from build123d import *

# Parameters (mm, degrees)
F0_W     = 273.05
F0_H     = 114.3
F1_DEPTH = 19.05
F2_R     = 25.4
F3_DEPTH = 25.4
F5_DEPTH = 25.4
F7_DEPTH = 25.4
F8_W     = 19.3382904482
F8_H     = 2.7599734166
F9_DEPTH = 25.4


# Not quite as in the source:
# - a feature names something its author has since deleted; it is built from what else it names


with BuildPart() as f1:
    # F0 (on Front) → F1 (new body)
    with BuildSketch(Plane.XZ):
        with Locations((136.525, 57.15)):
            Rectangle(F0_W, F0_H)
    extrude(amount=F1_DEPTH)

    # F2 (on face) → F3 (cut)
    with BuildSketch(Plane.XZ.offset(19.05)):
        with Locations((50.8, 47.625)):
            Circle(F2_R)
        with Locations((222.25, 47.625)):
            Circle(F2_R)
    extrude(amount=-F3_DEPTH, mode=Mode.SUBTRACT)

    # F4 (on face) → F5 (cut)
    with BuildSketch(Plane.XZ.offset(19.05)):
        with BuildLine():
            Line((200.0185036906, 35.3400265834), (73.0314963094, 35.3400265834))
            ThreePointArc((73.0314963094, 35.3400265834), (68.4136636998, 29.3242117364), (62.225616864, 24.9398665581))
            Line((62.225616864, 24.9398665581), (210.824383136, 24.9398665581))
            ThreePointArc((210.824383136, 24.9398665581), (204.6363363002, 29.3242117364), (200.0185036906, 35.3400265834))
        make_face()
    extrude(amount=-F5_DEPTH, mode=Mode.SUBTRACT)

    # F6 (on face) → F7 (cut)
    with BuildSketch(Plane.XZ.offset(19.05)):
        with BuildLine():
            Line((177.8, 114.3), (95.25, 114.3))
            Line((95.25, 114.3), (95.25, 49.53))
            ThreePointArc((95.25, 49.53), (98.597769491, 41.447769491), (106.68, 38.1))
            Line((106.68, 38.1), (166.37, 38.1))
            ThreePointArc((166.37, 38.1), (174.452230509, 41.447769491), (177.8, 49.53))
            Line((177.8, 49.53), (177.8, 114.3))
        make_face()
    extrude(amount=-F7_DEPTH, mode=Mode.SUBTRACT)

    # F8 (on face) → F9 (cut)
    with BuildSketch(Plane.XZ.offset(19.05)):
        with Locations((156.7008547759, 36.7200132917)):
            Rectangle(F8_W, F8_H)
    extrude(amount=-F9_DEPTH, mode=Mode.SUBTRACT)


solid = f1.part
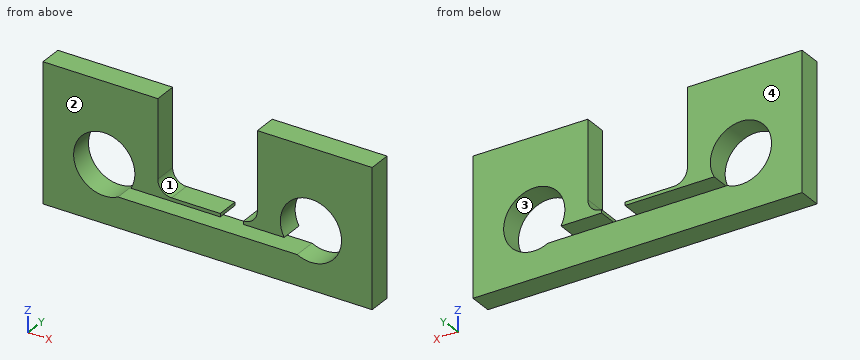
Design review of the part built by this model. Coordinates are the model's own, in mm. Face numbers are marked on the shaded views. A direction names the side the tool comes from. Give positions to 0.01 mm unless a question says otherwise; leave off trailing zeros. Write each loop counter-clockwise with the first axis right and the second up, starting at its lowest first coordinate (ties: lowest second). Pieces come first, ordered by that corner, then holes. Notation, with made-up numbers: M -32,22.25 L -2,22.25 A13 ccw -2,41.25 Z; hole C -23,5 d11. An arc over 180 degrees is marked long. Return JSON: item names as keys, results as strings. Group by question number.
Item 1: The part is to be moulded in two halves that separate along X. For the marked faces 3 and 4, say which applies: pulls with the +X half, pulls with the -X half, needs draft (parallel to the pull), parting line crosses it, or undercut.
Item 2: Wall thickness on line 1 along Z through (x, y) = (50.8, -4.5) (3 decimals); line 2 along X through (y, z) = (-12, 98); line 3 along X through (y, z) = (-17.25, 38): over which ranges is each line inside the solid? List them lowest first.
Item 3: Take a section at B-B (z = 84). Give the boundary of the cut face in (x, y).
Item 4: Tool access review of the marked faces 1 and 2: name each direction out of +Z, -Z, +X, -X, +Y, -Y from which nothing blocks a thin tool from reaching the whole face with its end or side.
Item 5: Clearance check with a flat-ended pin moving along its axis: pin 1 Ø10 at (y, z) = (-3.5, 80.5) entering from -X. State where the tip first meets the part, or that it passes through.
Item 6: Take a section at A-A (x = 86). Give the boundary of the cut face in (y, z), plus the area to 3 significant figures.
Return value:
{
 "1": {"face 3": "undercut", "face 4": "needs draft"},
 "2": {"line 1": "z = 0 to 22.225, 73.025 to 114.3", "line 2": "x = 0 to 95.25, 177.8 to 273.05", "line 3": "x = 0 to 27.29, 74.31 to 147.03, 166.37 to 198.74, 245.76 to 273.05"},
 "3": {"outline": "M 0,-19.05 L 95.25,-19.05 L 95.25,0 L 0,0 Z; M 177.8,-19.05 L 273.05,-19.05 L 273.05,0 L 177.8,0 Z"},
 "4": {"face 1": "+Z, +Y, -Y", "face 2": "+Z, -Z, +X, -X, -Y"},
 "5": {"pin 1": "stops at x = 0"},
 "6": {"outline": "M -19.05,0 L 0,0 L 0,24.94 L -19.05,24.94 Z; M -19.05,35.34 L 0,35.34 L 0,114.3 L -19.05,114.3 Z", "area": "1,980 mm2"}
}
